```python
from build123d import *

# Parameters (mm, degrees)
SKETCH3_R           = 37.2
BOSS_EXTRUDE1_DEPTH = 10
SKETCH4_R           = 36.2
CUT_EXTRUDE1_DEPTH  = 9
SKETCH5_R           = 30
CUT_EXTRUDE2_DEPTH  = 9
SKETCH6_R           = 58
SKETCH6_R_2         = 37.2
BOSS_EXTRUDE2_DEPTH = 4
SKETCH7_R           = 47.8
SKETCH7_R_2         = 46.5
BOSS_EXTRUDE3_DEPTH = 3


with BuildPart() as part:
    # Sketch3 → Boss-Extrude1 (new body)
    with BuildSketch(Plane(origin=(0, 0, 0), x_dir=(1, 0, 0), z_dir=(0, 1, 0))):
        with Locations(Location((0, 0, 0), (0, 0, 270))):
            Circle(SKETCH3_R)
    extrude(amount=BOSS_EXTRUDE1_DEPTH)

    # Sketch4 → Cut-Extrude1 (cut)
    with BuildSketch(Plane(origin=(0, 10, 0), x_dir=(1, 0, 0), z_dir=(0, 1, 0))):
        with Locations(Location((0, 0, 0), (0, 0, 270))):
            Circle(SKETCH4_R)
    extrude(amount=-CUT_EXTRUDE1_DEPTH, mode=Mode.SUBTRACT)

    # Sketch5 → Cut-Extrude2 (cut)
    with BuildSketch(Plane(origin=(0, 1, 0), x_dir=(1, 0, 0), z_dir=(0, 1, 0))):
        with Locations(Location((0, 0, 0), (0, 0, 270))):
            Circle(SKETCH5_R)
    extrude(amount=-CUT_EXTRUDE2_DEPTH, mode=Mode.SUBTRACT)

    # Sketch6 → Boss-Extrude2 (add)
    with BuildSketch(Plane(origin=(0, 6, 0), x_dir=(1, 0, 0), z_dir=(0, 1, 0))):
        with Locations(Location((0, 0, 0), (0, 0, 270))):
            Circle(SKETCH6_R)
        with Locations(Location((0, 0, 0), (0, 0, 270))):
            Circle(SKETCH6_R_2, mode=Mode.SUBTRACT)
    extrude(amount=BOSS_EXTRUDE2_DEPTH)

    # Sketch7 → Boss-Extrude3 (add)
    with BuildSketch(Plane.XZ.offset(-6)):
        with Locations(Location((0, 0, 0), (0, 0, 90))):
            Circle(SKETCH7_R)
        with Locations(Location((0, 0, 0), (0, 0, 270))):
            Circle(SKETCH7_R_2, mode=Mode.SUBTRACT)
    extrude(amount=BOSS_EXTRUDE3_DEPTH)


solid = part.part
```
The model under review builds one solid part; all positions refer to its coordinate system, in mm. A direction names the side the tool comes from. Give positions to 0.01 mm unless a question says otherwise; leave off trailing zeros. Write each loop counter-clockwise with the first axis right and the second up, starting at its lowest first coordinate (ties: lowest second). Pieces come first, ordered by that corner, then holes. Notation, with made-up numbers: M 11.5,-9.75 L 37.5,-9.75 A21 cw 37.5,-3.75 Z; hole C -15.5,68 d8. An arc over 180 degrees is marked long. Answer in a Markdown table with one row per item.
Item 1: Tool access review of faces 1 (the face through (17, 0, -25)), 2 (the face through (46.1, 4.5, 6.1)), 3 (the face through (27, 1, -14)): name each direction out of +Z, -Z, +X, -X, +Y, -Y from which nothing blocks a thin tool from reaching the whole face with its end or side.
Check sheet entries:
| item | result |
|---|---|
| face 1 | +Z, -Z, +X, -X, -Y |
| face 2 | -Y |
| face 3 | +Y |
Item 2: Add section A-A on x = 0. Give the boundary of the cut face in (y, z).
Check sheet entries:
| item | result |
|---|---|
| outline | M 0,-37.2 L 6,-37.2 L 6,-46.5 L 3,-46.5 L 3,-47.8 L 6,-47.8 L 6,-58 L 10,-58 L 10,-36.2 L 1,-36.2 L 1,-30 L 0,-30 Z; M 0,30 L 1,30 L 1,36.2 L 10,36.2 L 10,58 L 6,58 L 6,47.8 L 3,47.8 L 3,46.5 L 6,46.5 L 6,37.2 L 0,37.2 Z |
Item 3: For P1, Ø1.5, axis at y = 7.5, z = -6.5, coming from the +X side; P2, Ø3, axis at x = -35, y = 2.5, coming from the +Z side; P3, Ø1, axis at x = 16, y = 1.5, coming from the -Z side, all flat-tipped, find the tip position at first contact; note any pin that passes through.
Check sheet entries:
| item | result |
|---|---|
| P1 | x = 57.71 |
| P2 | z = 34.01 |
| P3 | z = -33.82 |
Item 4: Add section B-B on z = 0. Give the boundary of the cut face in (x, y).
Check sheet entries:
| item | result |
|---|---|
| outline | M -58,6 L -47.8,6 L -47.8,3 L -46.5,3 L -46.5,6 L -37.2,6 L -37.2,0 L -30,0 L -30,1 L -36.2,1 L -36.2,10 L -58,10 Z; M 30,0 L 37.2,0 L 37.2,6 L 46.5,6 L 46.5,3 L 47.8,3 L 47.8,6 L 58,6 L 58,10 L 36.2,10 L 36.2,1 L 30,1 Z |
Item 5: Draft analysis for pull direction Z (two halves, no side actions). For faces 4 (the face through (10.87, 5.56, 34.53)), 5 (the face through (48, 6, 8)), 6 (the face through (1.32, 0.51, -29.97)), 7 (the face through (-22.21, 7.97, 53.58)), state which applies: +Z half, -Z half, draft (parallel to the pull), parting line (faces both ways), or undercut.
Check sheet entries:
| item | result |
|---|---|
| face 4 | undercut |
| face 5 | draft |
| face 6 | undercut |
| face 7 | parting line |
Item 6: Add section C-C on z = 43.5. Give the boundary of the cut face in (x, y).
Check sheet entries:
| item | result |
|---|---|
| outline | M -38.36,6 L -19.81,6 L -19.81,3 L -16.43,3 L -16.43,6 L 16.43,6 L 16.43,3 L 19.81,3 L 19.81,6 L 38.36,6 L 38.36,10 L -38.36,10 Z |
Item 7: For line 1 along X through (y, z) = (5, 0); line 2 along X through (y, z) = (7.25, 0); line 3 along X through (y, z) = (0.6, 0), list the stretches that pass through material, from the lowest coordinate up.
Check sheet entries:
| item | result |
|---|---|
| line 1 | -47.8 to -46.5, -37.2 to -36.2, 36.2 to 37.2, 46.5 to 47.8 |
| line 2 | -58 to -36.2, 36.2 to 58 |
| line 3 | -37.2 to -30, 30 to 37.2 |
